```python
from build123d import *

# Parameters (mm, degrees)
SKETCH_1_W          = 15
SKETCH_1_H          = 15
SKETCH_1_W_2        = 13
SKETCH_1_H_2        = 13
EXTRUDE_1_DEPTH     = 460
SKETCH_2_R          = 1.45
CUT_EXTRUDE_1_DEPTH = 461.305605006
SKETCH_3_R          = 1.45
CUT_EXTRUDE_2_DEPTH = 461.305605006


with BuildPart() as part:
    # 草图1 → 拉伸-薄壁1 (new body)
    with BuildSketch(Plane(origin=(0, 0, 0), x_dir=(1, 0, 0), z_dir=(0, 1, 0))):
        Rectangle(SKETCH_1_W, SKETCH_1_H)
        Rectangle(SKETCH_1_W_2, SKETCH_1_H_2, mode=Mode.SUBTRACT)
    extrude(amount=EXTRUDE_1_DEPTH)

    # 草图2 → 切除-拉伸1 (cut, through all)
    with BuildSketch(Plane.XY.offset(7.5)):
        with Locations((0, 7.5)):
            Circle(SKETCH_2_R)
        with Locations((0, 27.5)):
            Circle(SKETCH_2_R)
        with Locations(Location((0, 432.5, 0), (0, 0, 180))):
            Circle(SKETCH_2_R)
        with Locations(Location((0, 452.5, 0), (0, 0, 180))):
            Circle(SKETCH_2_R)
        with Locations((0, 65)):
            Circle(SKETCH_2_R)
        with Locations((0, 85)):
            Circle(SKETCH_2_R)
        with Locations((0, 125)):
            Circle(SKETCH_2_R)
        with Locations((0, 145)):
            Circle(SKETCH_2_R)
        with Locations(Location((0, 315, 0), (0, 0, 180))):
            Circle(SKETCH_2_R)
        with Locations(Location((0, 335, 0), (0, 0, 180))):
            Circle(SKETCH_2_R)
        with Locations(Location((0, 375, 0), (0, 0, 180))):
            Circle(SKETCH_2_R)
        with Locations(Location((0, 395, 0), (0, 0, 180))):
            Circle(SKETCH_2_R)
        with Locations((0, 185)):
            Circle(SKETCH_2_R)
        with Locations(Location((0, 275, 0), (0, 0, 180))):
            Circle(SKETCH_2_R)
    extrude(amount=-CUT_EXTRUDE_1_DEPTH, mode=Mode.SUBTRACT)

    # 草图3 → 切除-拉伸2 (cut, through all)
    with BuildSketch(Plane(origin=(7.5, 0, 0), x_dir=(0, 0, -1), z_dir=(1, 0, 0))):
        with Locations((0, 152.5)):
            Circle(SKETCH_3_R)
        with Locations((0, 172.5)):
            Circle(SKETCH_3_R)
        with Locations((0, 287.5)):
            Circle(SKETCH_3_R)
        with Locations((0, 307.5)):
            Circle(SKETCH_3_R)
        with Locations((0, 192.5)):
            Circle(SKETCH_3_R)
        with Locations((0, 267.5)):
            Circle(SKETCH_3_R)
    extrude(amount=-CUT_EXTRUDE_2_DEPTH, mode=Mode.SUBTRACT)


solid = part.part
```
Can you work these out from the model? Positions are in its coordinate system, mm. A direction names the side the tool comes from. Round coordinates to 2 decimals unless told otherwise and drop trailing zeros. Loops run counter-clockwise (first coordinate to the right, second up) from the corner with the lowest first, then second, coordinate; pieces in that order, holes last. Notation, with made-up numbers: (76.5, -37) -> (90.5, -37) arc R20 cw to (90.5, -11) -> close; hole circle Ø5 at (38.5, 81). An arc over 180 degrees is marked (long way). Answer in a Markdown table with one row per item.
Item 1: If I drill on probe 1 along X at (y, z) = (185, -7.2); probe 2 along X at (y, z) = (325.5, -2.5), over which ranges is the centre line in solid material (lowest first)?
Answer block:
| item | result |
|---|---|
| probe 1 | -7.5 to -1.45, 1.45 to 7.5 |
| probe 2 | -7.5 to -6.5, 6.5 to 7.5 |
Item 2: On a 3-axis mill with a long thin cutter (end or side, diameter ignored), from which of +Z, -Z, +X, -X, +Y, -Y can I reach the whole of each face in a straight line? I mean faces 4 (the flat face through (0, 227, -6.5)), 5 (the flat face through (0, 227, -7.5)). Say none if no direction works.
Answer block:
| item | result |
|---|---|
| face 4 | +Y, -Y |
| face 5 | -Z, +X, -X, +Y, -Y |
Item 3: Suppose I cut it at A-A, the plane y = 366.5. List the corners of the cut face in (x, z) for me.
Answer block:
| item | result |
|---|---|
| outline | (-7.5, -7.5) -> (7.5, -7.5) -> (7.5, 7.5) -> (-7.5, 7.5) -> close; hole (-6.5, -6.5) -> (6.5, -6.5) -> (6.5, 6.5) -> (-6.5, 6.5) -> close |
Item 4: We'd pull the mould along X, two halves only. Please class faces 1 (the flat face through (-7.5, 227, 0)), 2 (the flat face through (-6.5, 227, 0)), 3 (the flat face through (0, 227, 7.5)): released by +X, released by -X, zero draft, split by the parting line, or undercut.
Answer block:
| item | result |
|---|---|
| face 1 | released by -X |
| face 2 | undercut |
| face 3 | zero draft |
Item 5: Will this pin go through, and if not, where does the flat tip stop? P1, Ø4.5, axis at x = 0, y = 185, coming from the +Z side.
Answer block:
| item | result |
|---|---|
| P1 | z = 7.5 |
